```python
from build123d import *

# Parameters (mm, degrees)
SKETCH1_R           = 4.7625
SKETCH1_R_2         = 3.175
BOSS_EXTRUDE1_DEPTH = 8.3312
BOSS_EXTRUDE2_DEPTH = 8.3312
SKETCH3_R           = 2.0875
SKETCH3_R_2         = 1.5875
BOSS_EXTRUDE3_DEPTH = 8.3312
SKETCH4_R           = 2.0875
BOSS_EXTRUDE4_DEPTH = 0.001
SKETCH5_R           = 1.78
SKETCH5_R_2         = 1.28
BOSS_EXTRUDE5_DEPTH = 11.5062
SKETCH6_R           = 10.258070852
CUT_EXTRUDE1_DEPTH  = 8.3312


with BuildPart() as part:
    # Sketch1 → Boss-Extrude1 (new body)
    with BuildSketch(Plane(origin=(0, 0, 0), x_dir=(1, 0, 0), z_dir=(0, 1, 0))):
        with Locations(Location((0, 0, 0), (0, 0, 270))):
            Circle(SKETCH1_R)
        with Locations(Location((0, 0, 0), (0, 0, 270))):
            Circle(SKETCH1_R_2, mode=Mode.SUBTRACT)
    extrude(amount=BOSS_EXTRUDE1_DEPTH)

    # Sketch2 → Boss-Extrude2 (add)
    with BuildSketch(Plane(origin=(0, 8.3312, 0), x_dir=(1, 0, 0), z_dir=(0, 1, 0))):
        Polygon((5.65061043, 0), (2.825305215, 4.893572179), (-2.825305215, 4.893572179), (-5.65061043, 0), (-2.825305215, -4.893572179), (2.825305215, -4.893572179), align=None)
    extrude(amount=BOSS_EXTRUDE2_DEPTH)

    # Sketch3 → Boss-Extrude3 (add)
    with BuildSketch(Plane(origin=(0, 16.6624, 0), x_dir=(1, 0, 0), z_dir=(0, 1, 0))):
        with Locations(Location((0, 0, 0), (0, 0, 270))):
            Circle(SKETCH3_R)
        with Locations(Location((0, 0, 0), (0, 0, 270))):
            Circle(SKETCH3_R_2, mode=Mode.SUBTRACT)
    extrude(amount=BOSS_EXTRUDE3_DEPTH)

    # Sketch4 → Boss-Extrude4 (add)
    with BuildSketch(Plane(origin=(0, 24.9936, 0), x_dir=(1, 0, 0), z_dir=(0, 1, 0))):
        with Locations(Location((0, 0, 0), (0, 0, 270))):
            Circle(SKETCH4_R)
    extrude(amount=BOSS_EXTRUDE4_DEPTH)

    # Sketch5 → Boss-Extrude5 (add)
    with BuildSketch(Plane.XY):
        with Locations(Location((0, 22.9946, 0), (0, 0, 180))):
            Circle(SKETCH5_R)
        with Locations(Location((0, 22.9946, 0), (0, 0, 180))):
            Circle(SKETCH5_R_2, mode=Mode.SUBTRACT)
    extrude(amount=BOSS_EXTRUDE5_DEPTH)

    # Sketch6 → Cut-Extrude1 (cut)
    with BuildSketch(Plane.XZ):
        Circle(SKETCH6_R)
    extrude(amount=-CUT_EXTRUDE1_DEPTH, mode=Mode.SUBTRACT)


solid = part.part
```
For this review, take the finished solid that the model builds, in its own axes (mm). A direction names the side the tool comes from. Round coordinates to 2 decimals unless told otherwise and drop trailing zeros. Loops run counter-clockwise (first coordinate to the right, second up) from the corner with the lowest first, then second, coordinate; pieces in that order, holes last.
(1) Wall thickness on line 1 along Y through (x, z) = (4.5, 1); line 2 along X through (y, z) = (22.5, 3.25); line 3 along X through (y, z) = (21.5, 8.25): over which ranges is each line inside the solid? List them lowest first.
Returned:
line 1: y = 8.33 to 16.66
line 2: x = -1.71 to -1.18, 1.18 to 1.71
line 3: x = -0.97 to 0.97
(2) Tool access review of faces 4 (the cylindrical face through (0.07, 20.77, -1.586)), 5 (the flat face through (-4.26, 12.44, 2.41)), 6 (the cylindrical face through (-0.821, 24.574, 6.225)), 7 (the flat face through (0, 12, -4.894)), 8 (the flat face through (0, 12, 4.894)): name each direction out of +Z, -Z, +X, -X, +Y, -Y from which nothing blocks a thin tool from reaching the whole face with its end or side.
Returned:
face 4: none
face 5: +Z, -X, +Y, -Y
face 6: +Z
face 7: -Z, +X, -X, +Y, -Y
face 8: +Z, +X, -X, -Y
(3) We need section C-C (y = 11.5). Give the boundary of the cut face in (x, z), plus the area to 3 significant figures.
Returned:
outline: (-5.65, 0) - (-2.83, -4.89) - (2.83, -4.89) - (5.65, 0) - (2.83, 4.89) - (-2.83, 4.89) - close
area: 83.0 mm2
(4) We need section A-A (x = 0). Give the boundary of the cut face in (y, z), plus the area to 3 significant figures.
Returned:
outline: (8.33, -4.89) - (16.66, -4.89) - (16.66, -2.09) - (24.99, -2.09) - (24.99, 2.09) - (24.77, 2.09) - (24.77, 11.51) - (24.27, 11.51) - (24.27, 2.09) - (21.71, 2.09) - (21.71, 11.51) - (21.21, 11.51) - (21.21, 2.09) - (16.66, 2.09) - (16.66, 4.89) - (8.33, 4.89) - close; hole (16.66, -1.59) - (24.99, -1.59) - (24.99, 1.59) - (24.77, 1.59) - (24.77, 0) - (24.27, 0) - (24.27, 1.59) - (21.71, 1.59) - (21.71, 0) - (21.21, 0) - (21.21, 1.59) - (16.66, 1.59) - close
area: 101 mm2
(5) Clearance check with flat-ended pins moving along their axes: P1, Ø2, axis at x = 0, y = 22.99, coming from the +Z side; P2, Ø4, axis at x = 2, z = 7.5, coming from the +Y side; P3, Ø3.5, axis at x = 0, y = 22.99, coming from the +Z side; P4, Ø1, axis at x = -0.5, y = 23.5, coming from the -Z side. State where each tip first meets the part, or that it passes through.
Returned:
P1: stops at z = 2.09
P2: stops at y = 24.77
P3: stops at z = 11.51
P4: stops at z = -2.09
(6) We need section D-D (x = -4.5). Give the boundary of the cut face in (y, z), plus the area to 3 significant figures.
Returned:
outline: (8.33, -1.99) - (16.66, -1.99) - (16.66, 1.99) - (8.33, 1.99) - close
area: 33.2 mm2
(7) Mouldability with a two-part tool opening along Y and no side actions: class faces 1 (the flat face through (0, 8.331, 0)), 2 (the cylindrical face through (-1.22, 22.61, 0.61)), 3 (the flat face through (-4.22, 12.44, -2.48)) as released by +Y, released by -Y, zero draft, split by the parting line, or undercut.
Returned:
face 1: released by -Y
face 2: undercut
face 3: zero draft
